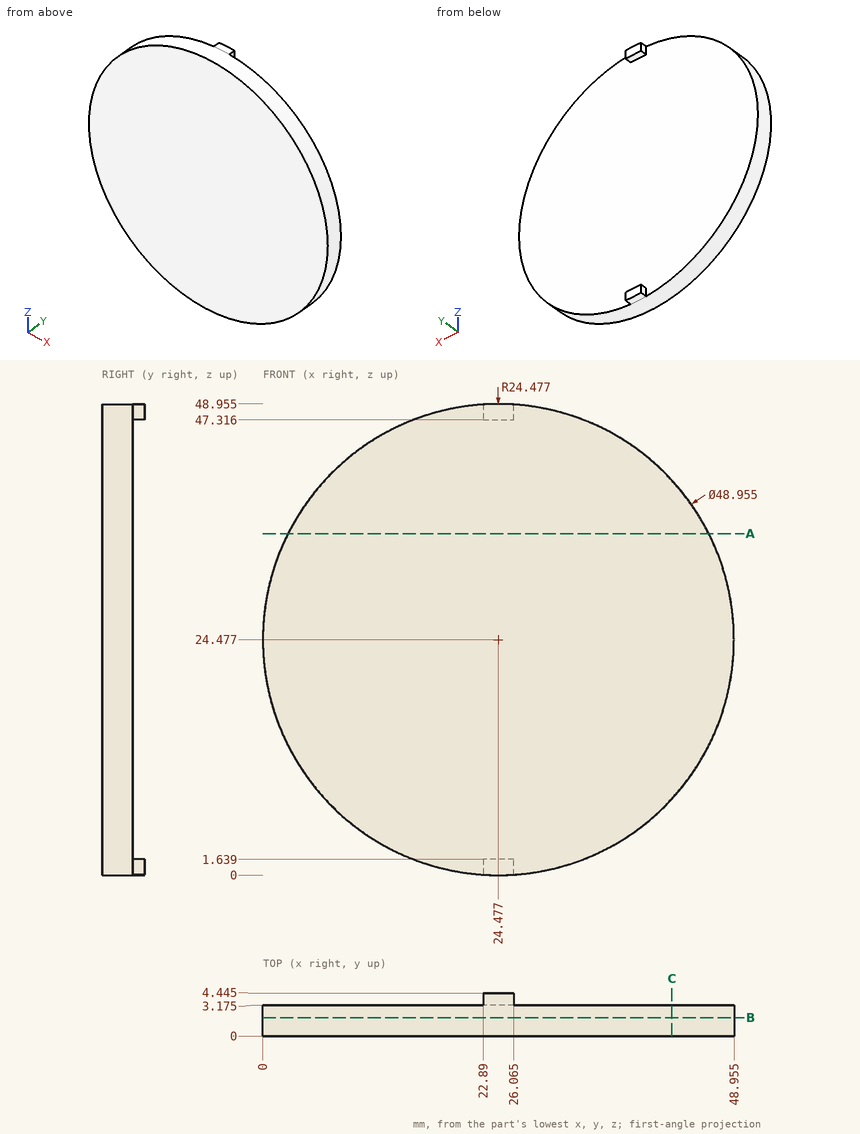
Geometry check sheet. Reference: drawing and pictorial views, mm from the part's lowest x, y, z. Round coordinates to 2 decimals unless told otherwise and drop trailing zeros. Write each loop counter-clockwise with the first axis right and the second up, starting at its lowest first coordinate (ties: lowest second). Pieces come first, ordered by that corner, then holes. Notation, with made-up numbers: (46, 54.25) -> (52, 54.25) arc R30 ccw to (52, 91.25) -> close; hole circle Ø6 at (70, 14). An arc over 180 degrees is marked (long way). Answer as CSV lines item,"result". Start each with the question number.
1) Section check B-B on y = 1.9. Enter the section's corners in (x, z) (1 decimal), and give its area (3 significant figures).
2) Go/stop test with flat-tipped pins: P1, Ø0.6, axis at y = 4, z = 1, coming from the +X side (1 decimal); P2, Ø2, axis at y = 1.5, z = 36.5, coming from the -X side; P3, Ø1, axis at y = 4, z = 48, coming from the -X side. Record where each tip stops, or that it passes through.
3) Section check C-C on x = 42.5. Enter the section's corners in (y, z) (1 decimal), and give its area (3 significant figures).
4) Material ranges on line 1 (Y direction, x = 45.5, z = 35) (1 decimal); line 2 (X direction, y = 0.5, z = 29); line 3 (Z direction, x = 39, y = 1.6) (1 decimal), recorded low to high. Write a range as from..to.
5) Section check A-A on z = 35.5. Enter the section's corners in (x, y) (1 decimal), and give its area (3 significant figures).
Found:
1,outline,"circle Ø49 at (24.5, 24.5)"
1,area,"1,880 mm^2"
2,P1,"stops at x = 26.1"
2,P2,"stops at x = 2.62"
2,P3,"stops at x = 22.89"
3,outline,"(0, 7.9) -> (3.2, 7.9) -> (3.2, 41) -> (0, 41) -> close"
3,area,"105 mm^2"
4,line 1,"y = 0..3.2"
4,line 2,"x = 0.42..48.53"
4,line 3,"z = 4.8..44.2"
5,outline,"(2.6, 0) -> (46.3, 0) -> (46.3, 3.2) -> (2.6, 3.2) -> close"
5,area,"139 mm^2"
